Check sheet for the modelled part. Datum: model origin and axes. Units: mm. Face numbers are marked on the shaded views. A direction names the side the tool comes from. Round coordinates to 2 decimals unless told otherwise and drop trailing zeros. Write each loop counter-clockwise with the first axis right and the second up, starting at its lowest first coordinate (ties: lowest second). Pieces come first, ordered by that corner, then holes. Notation, with made-up numbers: M 4,71 L 35,71 A18 cw 35,103 Z; hole C 84.25,-15 d2. An arc over 180 degrees is marked long. Put each result on its own line as item: value.
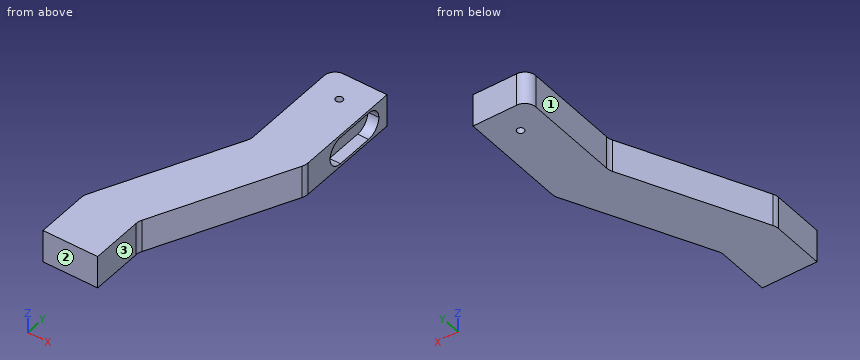
```python
from build123d import *

# Parameters (mm, degrees)
F1_DEPTH    = 30
F2_W        = 60
F2_H        = 25
F3_DEPTH    = 10
F4_R        = 10
F5_R        = 3.2639
F6_DEPTH    = 30.001
F7_T1_DEPTH = 30
F7_T3_DEPTH = 10
F7_T5_DEPTH = 41.75
F7_T7_DEPTH = 44.4507439359


# Not quite as in the source:
# - a fillet or chamfer that OpenCascade refuses, or shapes differently, is made with other operations: its cross-section is extruded or revolved along the edge and cut away or added


with BuildPart() as f1:
    # F0 (on Top) → F1 (new body)
    with BuildSketch(Plane.XY):
        Polygon((-25, -100), (-25, -150), (25, -150), (25, -100), (85, 25), (85, 125), (35, 125), (35, 25), align=None)
    extrude(amount=F1_DEPTH)

    # F2 (on face) → F3 (cut)
    with BuildSketch(Plane.YZ.offset(85)):
        with Locations((85, 15)):
            Rectangle(F2_W, F2_H)
    extrude(amount=-F3_DEPTH, mode=Mode.SUBTRACT)

    # F4
    f4_edges = [f1.edges().sort_by_distance(p)[0] for p in [
        (35, 125, 15),
    ]]
    fillet(f4_edges, radius=F4_R)

    # F5 (on face) → F6 (cut, through all)
    with BuildSketch(Plane.XY.offset(30)):
        with Locations((60, 100)):
            Circle(F5_R)
    extrude(amount=-F6_DEPTH, mode=Mode.SUBTRACT)

    # F7: fillet of radius 12.7 on 8 edges, made by hand

    # F7_s2 → F7_t1 (join)
    with BuildSketch(Plane.XY):
        with BuildLine():
            ThreePointArc((26.2506571702, -97.3944642288), (25.3166108448, -100.0720513739), (25, -102.8901487872))
            Line((25, -102.8901487872), (25, -100))
            Line((25, -100), (26.2506571702, -97.3944642288))
        make_face()
        with BuildLine():
            ThreePointArc((35, 27.8901487872), (34.6833891552, 25.0720513739), (33.7493428298, 22.3944642288))
            Line((33.7493428298, 22.3944642288), (35, 25))
            Line((35, 25), (35, 27.8901487872))
        make_face()
    extrude(amount=F7_T1_DEPTH)

    # F7_s4 → F7_t3 (join)
    with BuildSketch(Plane.YZ.offset(75)):
        with BuildLine():
            ThreePointArc((102.3, 27.5), (111.2802561211, 23.7802561211), (115, 14.8))
            Line((115, 14.8), (115, 27.5))
            Line((115, 27.5), (102.3, 27.5))
        make_face()
        with BuildLine():
            ThreePointArc((115, 15.2), (111.2802561211, 6.2197438789), (102.3, 2.5))
            Line((102.3, 2.5), (115, 2.5))
            Line((115, 2.5), (115, 15.2))
        make_face()
    extrude(amount=F7_T3_DEPTH)

    # F7_s6 → F7_t5 (join)
    with BuildSketch(Plane.YZ.offset(43.25)):
        with BuildLine():
            ThreePointArc((67.7, 27.5), (58.7197438789, 23.7802561211), (55, 14.8))
            Line((55, 14.8), (55, 27.5))
            Line((55, 27.5), (67.7, 27.5))
        make_face()
        with BuildLine():
            ThreePointArc((67.7, 2.5), (58.7197438789, 6.2197438789), (55, 15.2))
            Line((55, 15.2), (55, 2.5))
            Line((55, 2.5), (67.7, 2.5))
        make_face()
    extrude(amount=F7_T5_DEPTH)

    # F7_s8 → F7_t7 (cut)
    with BuildSketch(Plane.XY.offset(-7.2253719679)):
        with BuildLine():
            ThreePointArc((85, 27.8901487872), (84.6833891552, 25.0720513739), (83.7493428298, 22.3944642288))
            Line((83.7493428298, 22.3944642288), (85, 25))
            Line((85, 25), (85, 27.8901487872))
        make_face()
        with BuildLine():
            ThreePointArc((-23.7493428298, -97.3944642288), (-24.6833891552, -100.0720513739), (-25, -102.8901487872))
            Line((-25, -102.8901487872), (-25, -100))
            Line((-25, -100), (-23.7493428298, -97.3944642288))
        make_face()
    extrude(amount=F7_T7_DEPTH, mode=Mode.SUBTRACT)


solid = f1.part
```
1. Cross-section at D-D (z = 10). Enter the section's corners in (x, y), then the cut area to 3 significant figures.
Computed values:
outline: M -25,-150 L 25,-150 L 25,-102.89 A12.7 cw 26.25,-97.39 L 83.75,22.39 A12.7 ccw 85,27.89 L 85,56.11 L 75,56.11 L 75,113.89 L 85,113.89 L 85,125 L 45,125 A10 ccw 35,115 L 35,27.89 A12.7 cw 33.75,22.39 L -23.75,-97.39 A12.7 ccw -25,-102.89 Z; hole C 60,100 d6.53
area: 13,100 mm2
2. Cross-section at C-C (x = 60). Enter the section's corners in (y, z), then the cut area to 3 significant figures.
Computed values:
outline: M -27.08,0 L 96.74,0 L 96.74,30 L -27.08,30 Z; M 103.26,0 L 125,0 L 125,30 L 103.26,30 Z
area: 4,370 mm2
3. Cross-section at B-B (y = 84). Enter the section's corners in (x, z), then the cut area to 3 significant figures.
Computed values:
outline: M 35,0 L 85,0 L 85,2.5 L 75,2.5 L 75,27.5 L 85,27.5 L 85,30 L 35,30 Z
area: 1,250 mm2
4. Cross-section at A-A (z = 20.5). Enter the section's corners in (x, y), then the cut area to 3 significant figures.
Computed values:
outline: M -25,-150 L 25,-150 L 25,-102.89 A12.7 cw 26.25,-97.39 L 83.75,22.39 A12.7 ccw 85,27.89 L 85,56.35 L 75,56.35 L 75,113.65 L 85,113.65 L 85,125 L 45,125 A10 ccw 35,115 L 35,27.89 A12.7 cw 33.75,22.39 L -23.75,-97.39 A12.7 ccw -25,-102.89 Z; hole C 60,100 d6.53
area: 13,100 mm2
5. Scan lines: probe 1 along Z at (x, y) = (76, 87); probe 2 along X at (y, z) = (70.5, 21); probe 3 along Y at (x, z) = (60, 16.5). Record each from-to range of solid material in increasing order.
Computed values:
probe 1: z = 0 to 2.5, 27.5 to 30
probe 2: x = 35 to 75
probe 3: y = -27.08 to 96.74, 103.26 to 125
6. Access from +Z, -Z, +X, -X, +Y, -Y to the whole of each face (thin tool, end or side, straight path). Record for the marked faces 1, 2 and 3.
Computed values:
face 1: +Z, -Z, -X, +Y
face 2: +Z, -Z, +X, -X, -Y
face 3: +Z, -Z, +X, -Y
7. Depth check by flat-ended pin: pin 1 Ø6 at (y, z) = (-76.5, 20) entering from -X; pin 2 Ø4 at (y, z) = (-33.5, 6) entering from +X; pin 3 Ø1 at (x, z) = (52.5, 7) entering from -Y; pin 4 Ø5 at (x, y) = (35, 91.5) entering from -Z. Enter the tip coordinate at first touch or a pass-through.
Computed values:
pin 1: stops at x = -15.16
pin 2: stops at x = 57.88
pin 3: stops at y = -43.75
pin 4: stops at z = 0
